For this review, take the finished solid that the model builds, in its own axes (mm). Coordinates: 2 decimals unless noted, no trailing zeros. Loops run counter-clockwise (first coordinate to the right, second up) from the corner with the lowest first, then second, coordinate; pieces in that order, holes last. Notation, with made-up numbers: (79.25, 29) - (93.25, 29) arc R19 cw to (93.25, 46) - close; hole circle Ø6 at (45, 35.5). An arc over 180 degrees is marked (long way). Answer as a JSON object with one key per item and string values. Group by question number.
Item 1: Clearance check with flat-ended pins moving along their axes: pin 1 (2 mm diameter, centred on y = 23, z = 3.5, fed in from +X); pin 2 (5 mm diameter, centred on x = 53, z = 4, fed in from +Y); pin 3 (3 mm diameter, centred on x = -71, z = 4, fed in from +Y); pin 4 (8 mm diameter, centred on x = 42, y = -18, fed in from -Z). State where each tip first meets the part, or that it passes through.
Item 2: To check wall thickness, follow line 1 (Y direction, x = 97, z = 3.5); line 2 (Y direction, x = 0.5, z = 1.25); line 3 (Y direction, x = 32.5, z = 7.75). State the ranges of each line that lie inside material, in increasing order.
Item 3: We need section A-A (z = 6.25). Give the boundary of the cut face in (x, y), then the cut area to 3 significant figures.
Item 4: We need section B-B (x = 44). Give the boundary of the cut face in (y, z), then the cut area to 3 significant figures.
Item 5: We need section C-C (y = 18). Give the boundary of the cut face in (x, z).
from build123d import *

# Parameters (mm, degrees)
F1_DEPTH = 9.906


# Not quite as in the source:
# - a feature names something its author has since deleted; it is built from what else it names


with BuildPart() as f1:
    # F0 (on Top) → F1 (new body)
    with BuildSketch(Plane.XY):
        with BuildLine():
            Line((-38.1069101836, -13.6540351038), (-87.8979010638, -13.6540351038))
            Line((-87.8979010638, -13.6540351038), (-87.8979010638, -40.5354308852))
            Line((-87.8979010638, -40.5354308852), (20.0543733488, -40.5354308852))
            Line((20.0543733488, -40.5354308852), (20.0543733488, -35.1623575424))
            ThreePointArc((20.0543733488, -35.1623575424), (-14.0401390689, -37.9663505394), (-38.1069101836, -13.6540351038))
        make_face()
        with BuildLine():
            ThreePointArc((30.0739874694, -27.0947329945), (25.3867048086, -31.5291055584), (20.0543733488, -35.1623575424))
            Line((20.0543733488, -35.1623575424), (20.0543733488, -40.5354308852))
            Line((20.0543733488, -40.5354308852), (108.3789337528, -40.5354308852))
            Line((108.3789337528, -40.5354308852), (108.3789337528, -27.0947329945))
            Line((108.3789337528, -27.0947329945), (30.0739874694, -27.0947329945))
        make_face()
        with BuildLine():
            Line((20.0543733488, -13.6540351038), (-38.1069101836, -13.6540351038))
            ThreePointArc((-38.1069101836, -13.6540351038), (-14.0401390689, -37.9663505394), (20.0543733488, -35.1623575424))
            Line((20.0543733488, -35.1623575424), (20.0543733488, -27.0947329945))
            Line((20.0543733488, -27.0947329945), (20.0543733488, -13.6540351038))
        make_face()
        with BuildLine():
            Line((20.0543733488, -27.0947329945), (20.0543733488, -35.1623575424))
            ThreePointArc((20.0543733488, -35.1623575424), (25.3867048086, -31.5291055584), (30.0739874694, -27.0947329945))
            Line((30.0739874694, -27.0947329945), (20.0543733488, -27.0947329945))
        make_face()
        with BuildLine():
            ThreePointArc((40.4792450319, 0), (-6.9292973534, 39.8817516734), (-38.1069101836, -13.6540351038))
            Line((-38.1069101836, -13.6540351038), (20.0543733488, -13.6540351038))
            Line((20.0543733488, -13.6540351038), (20.0543733488, -27.0947329945))
            Line((20.0543733488, -27.0947329945), (30.0739874694, -27.0947329945))
            ThreePointArc((30.0739874694, -27.0947329945), (37.7885008052, -14.5120117574), (40.4792450319, 0))
        make_face()
    extrude(amount=F1_DEPTH)


solid = f1.part
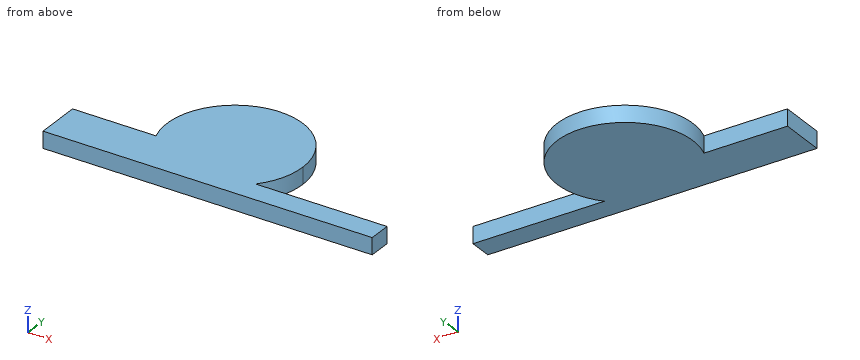
Check sheet entries:
{
 "1": {"pin 1": "stops at x = 33.98", "pin 2": "stops at y = -27.09", "pin 3": "stops at y = -13.65", "pin 4": "passes through"},
 "2": {"line 1": "y = -40.54 to -27.09", "line 2": "y = -40.54 to 40.48", "line 3": "y = -40.54 to -27.09, -24.13 to 24.13"},
 "3": {"outline": "(-87.9, -40.54) - (108.38, -40.54) - (108.38, -27.09) - (30.07, -27.09) arc R40.48 ccw (long way) to (-38.11, -13.65) - (-87.9, -13.65) - close", "area": "7,940 mm2"},
 "4": {"outline": "(-40.54, 0) - (-27.09, 0) - (-27.09, 9.91) - (-40.54, 9.91) - close", "area": "133 mm2"},
 "5": {"outline": "(-36.26, 0) - (36.26, 0) - (36.26, 9.91) - (-36.26, 9.91) - close"}
}
